```python
from build123d import *

# Parameters (mm, degrees)
SKETCH1_W           = 19
SKETCH1_H           = 68.229050279
BOSS_EXTRUDE1_DEPTH = 1000


with BuildPart() as part:
    # Sketch1 → Boss-Extrude1 (new body)
    with BuildSketch(Plane(origin=(0, 0, 0), x_dir=(0, 0, -1), z_dir=(1, 0, 0))):
        Polygon((0, 13.337988827), (0, 0), (50, 0), (53, 0), (72, 0), (75, 0), (500, 0), (500, 13.337988827), align=None)
        Polygon((53, 0), (50, 0), (50, -72), (53, -72), (53, -68.229050279), align=None)
        with Locations((62.5, -34.11452514)):
            Rectangle(SKETCH1_W, SKETCH1_H)
        Polygon((75, 0), (72, 0), (72, -68.229050279), (72, -72), (75, -72), align=None)
    extrude(amount=BOSS_EXTRUDE1_DEPTH)


solid = part.part
```
Can you work these out from the model? Positions are in its coordinate system, mm. A direction names the side the tool comes from. Coordinates: 2 decimals unless noted, no trailing zeros. Order: outer loops, then holes, each group sorted by start corner. A loop starts at its lowest first (then second) coordinate and runs counter-clockwise, first axis right, second up.
1. If we section it at C-C (y = -45): Please give me the cut outline in (x, z).
2. I'm going to push flat-ended pins straight in: pin 1 (1 mm diameter, centred on x = 492, z = -419.5, fed in from -Y); pin 2 (1.5 mm diameter, centred on x = 240, y = -56.5, fed in from +Z); pin 3 (3 mm diameter, centred on x = 647, y = -70.5, fed in from -Z). Where does each tip first touch, or does it pass through?
3. I need wall thicknesses on line 1 (Z direction, x = 706, y = -36.5); line 2 (Y direction, x = 397, z = -425). Which ranges of each line are inside material? Lowest first, please.
4. If we section it at A-A (x = 224): Please give me the cut outline in (y, z), then the cut area to 3 significant figures.
5. For faces 1 (the face through (493, -35, -50)), 2 (the face through (493, 0, -285)), 3 (the face through (493, 13.338, -253)), which set-ups out of +Z, -Z, +X, -X, +Y, -Y let a thin tool reach every point of the face, with its end or its side?
6. Thinking about a two-plate mould opening in Z: for faces 4 (the face through (1000, 2, -212)), 5 (the face through (493, -37, -75)), 6 (the face through (493, -68.229, -62)), which applies, +Z half, -Z half, draft (parallel to the pull), parting line (faces both ways), or undercut?
7. If we section it at B-B (z = -407): Please give me the cut outline in (x, y), then the cut area to 3 significant figures.
Entries:
1. outline: (0, -75) - (1000, -75) - (1000, -50) - (0, -50) - close
2. pin 1: stops at y = 0
2. pin 2: stops at z = -50
2. pin 3: stops at z = -75
3. line 1: z = -75 to -50
3. line 2: y = 0 to 13.34
4. outline: (-72, -75) - (0, -75) - (0, -500) - (13.34, -500) - (13.34, 0) - (0, 0) - (0, -50) - (-72, -50) - (-72, -53) - (-68.23, -53) - (-68.23, -72) - (-72, -72) - close
4. area: 8,400 mm2
5. face 1: +Z, +X, -X, -Y
5. face 2: -Z, +X, -X, -Y
5. face 3: +Z, -Z, +X, -X, +Y
6. face 4: draft
6. face 5: -Z half
6. face 6: undercut
7. outline: (0, 0) - (1000, 0) - (1000, 13.34) - (0, 13.34) - close
7. area: 13,300 mm2
